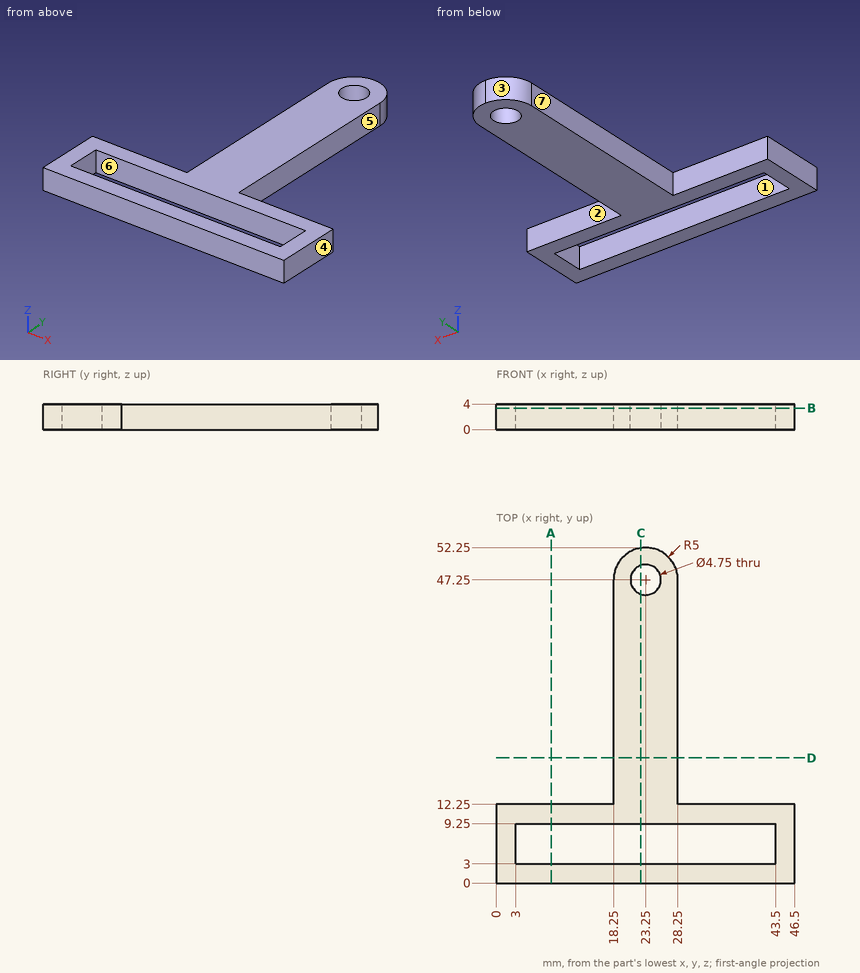
Print and shaded views of the part. All mm, measured from the part's lowest x, y and z. A direction names the side the tool comes from. Coordinates: 2 decimals unless noted, no trailing zeros. Write each loop counter-clockwise with the first axis right and the second up, starting at its lowest first coordinate (ties: lowest second). Pieces come first, ordered by that corner, then holes.
(1) Cut at B-B, the plane z = 3.35. Count the separate pieces of the cut face and the enclosed holes in it, and give its area (3 significant figures).
(2) Drill centre lines: probe 1 along Y at (x, z) = (23.25, 2.25) (3 decimals); probe 2 along Y at (x, z) = (31.5, 2.25); probe 3 along X at (y, z) = (16.5, 2.5). Where is each one in solid material? Low to high.
(3) Cut at A-A, the plane x = 8.5. List the corners of the cut face in (y, z), and give its area (3 significant figures).
(4) Two-plate mould, pull along X, no slides. Class the marked faces 1, 2 and 3: +X half, -X half, draft (parallel to the pull), parting line (faces both ways), or undercut.
(5) 3-axis set-ups, long thin cutter, end or side, ignore diameter. For the marked faces 4, 5, 6 and 7: which of +Z, -Z, +X, -X, +Y, -Y reach the whole face in a straight line?
(6) Flat gauge pins, fed straight in: pin 1 (1.2 mm diameter, centred on x = 19, z = 1, fed in from +Y); pin 2 (2 mm diameter, centred on x = 8.5, z = 2, fed in from +Y); pin 3 (4.5 mm diameter, centred on x = 23.25, y = 47.25, fed in from -Z); pin 4 (2 mm diameter, centred on y = 5, z = 1.5, fed in from -X). Where does each tip first touch, or does it go through?
(7) Cut at C-C, the plane x = 22.5. List the corners of the cut face in (y, z), and give its area (3 significant figures).
(8) Cut at D-D, the plane y = 19.5. List the corners of the cut face in (x, z).
Geometry says:
1. separate pieces: 1
1. enclosed holes: 2
1. area: 688 mm2
2. probe 1: y = 0 to 3, 9.25 to 44.875, 49.625 to 52.25
2. probe 2: y = 0 to 3, 9.25 to 12.25
2. probe 3: x = 18.25 to 28.25
3. outline: (0, 0) - (3, 0) - (3, 4) - (0, 4) - close; (9.25, 0) - (12.25, 0) - (12.25, 4) - (9.25, 4) - close
3. area: 24.0 mm2
4. face 1: undercut
4. face 2: draft
4. face 3: -X half
5. face 4: +Z, -Z, +X, +Y, -Y
5. face 5: +Z, -Z, +X, +Y
5. face 6: +Z, -Z
5. face 7: +Z, -Z, -X, +Y
6. pin 1: stops at y = 50.67
6. pin 2: stops at y = 12.25
6. pin 3: passes through
6. pin 4: stops at x = 0
7. outline: (0, 0) - (3, 0) - (3, 4) - (0, 4) - close; (9.25, 0) - (45, 0) - (45, 4) - (9.25, 4) - close; (49.5, 0) - (52.19, 0) - (52.19, 4) - (49.5, 4) - close
7. area: 166 mm2
8. outline: (18.25, 0) - (28.25, 0) - (28.25, 4) - (18.25, 4) - close
